```python
from build123d import *

# Parameters (mm, degrees)
SKETCH_1_R          = 2.75
EXTRUDE_1_DEPTH     = 3
FILLET_1_R          = 0.5
CUT_EXTRUDE_1_DEPTH = 2
SKETCH_3_R          = 1.5
EXTRUDE_2_DEPTH     = 8
CHAMFER_1_SIZE      = 0.2
FILLET_2_R          = 0.2


with BuildPart() as part:
    # 草图1 → 凸台-拉伸1 (new body)
    with BuildSketch(Plane.XY):
        Circle(SKETCH_1_R)
    extrude(amount=EXTRUDE_1_DEPTH)

    # 圆角1
    fillet_1_edges = [part.edges().sort_by_distance(p)[0] for p in [
        (-2.75, 0, 3),
    ]]
    fillet(fillet_1_edges, radius=FILLET_1_R)

    # 草图2 → 切除-拉伸1 (cut)
    with BuildSketch(Plane.XY.offset(3)):
        Polygon((1.558845727, 0), (0.779422863, 1.35), (-0.779422863, 1.35), (-1.558845727, 0), (-0.779422863, -1.35), (0.779422863, -1.35), align=None)
    extrude(amount=-CUT_EXTRUDE_1_DEPTH, mode=Mode.SUBTRACT)

    # 草图3 → 凸台-拉伸2 (add)
    with BuildSketch(Plane(origin=(0, 0, 0), x_dir=(-1, 0, 0), z_dir=(0, 0, -1))):
        Circle(SKETCH_3_R)
    extrude(amount=EXTRUDE_2_DEPTH)

    # 倒角1
    chamfer_1_edges = [part.edges().sort_by_distance(p)[0] for p in [
        (1.5, 0, -8),
    ]]
    chamfer(chamfer_1_edges, length=CHAMFER_1_SIZE)

    # 圆角2
    fillet_2_edges = [part.edges().sort_by_distance(p)[0] for p in [
        (-2.75, 0, 0),
    ]]
    fillet(fillet_2_edges, radius=FILLET_2_R)


solid = part.part
```
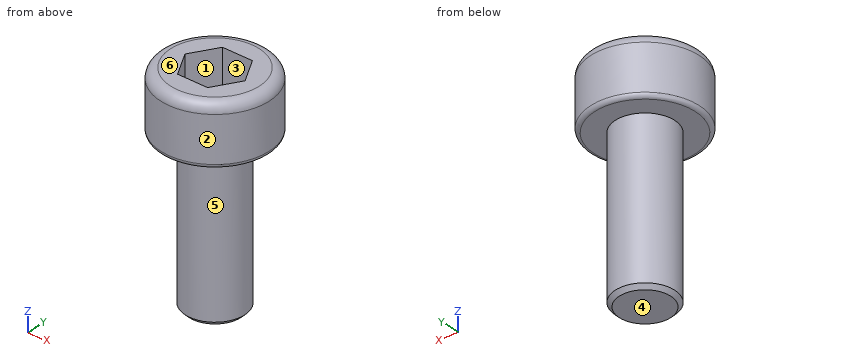
Input: part model. Units: mm. Frame: model coordinates. Face numbers are marked on the shaded views. A direction names the side the tool comes from. Coordinates: 2 decimals unless noted, no trailing zeros. Loops run counter-clockwise (first coordinate to the right, second up) from the corner with the lowest first, then second, coordinate; pieces in that order, holes last. Notation, with made-up numbers: M 3.25,20.25 L 34.25,20.25 A9 ccw 34.25,26.25 Z; hole C -19,24.25 d6. An arc over 180 degrees is marked long. Use a Markdown table: item, result. Add a question column.
1) Line query: L1, parallel to X at y = -0.75, z = -5.5; L2, parallel to Z at x = -0.9, y = -0.1. Output: solid intervals per line, ascending. Write a range as from..to.
2) Section A-A, the plane x = 0. Return the cut outline in (y, z), plus the area to 3 significant figures.
3) Section B-B, the plane z = -2. Return the cut outline in (x, y).
4) Draft query along X for the marked faces 1, 2, 3 and 4. Return one class per face: +X half, -X half, draft (parallel to the pull), parting line (faces both ways), or undercut.
5) Pin query (flat end, axial travel): P1, Ø1.7, axis at x = 0.5, z = 2, coming from the +Y side; P2, Ø0.5, axis at x = -0.5, z = 2, coming from the -Y side; P3, Ø2, axis at x = -1.5, z = -1.5, coming from the -Y side; P4, Ø1.5, axis at x = 0.5, z = -2.5, coming from the -Y side. Return the tip coordinate at first contact, or that it passes through.
6) Set-up query: the marked faces 5 and 6. Return all of +Z, -Z, +X, -X, +Y, -Y with unobstructed straight access to the full face (end or side cutting, diameter ignored); none if empty.
Answer below:
| question | item | result |
|---|---|---|
| 1 | L1 | -1.3..1.3 |
| 1 | L2 | -8..1 |
| 2 | outline | M -2.75,0.2 A0.2 ccw -2.55,0 L -1.5,0 L -1.5,-7.8 L -1.3,-8 L 1.3,-8 L 1.5,-7.8 L 1.5,0 L 2.55,0 A0.2 ccw 2.75,0.2 L 2.75,2.5 A0.5 ccw 2.25,3 L 1.35,3 L 1.35,1 L -1.35,1 L -1.35,3 L -2.25,3 A0.5 ccw -2.75,2.5 Z |
| 2 | area | 34.9 mm2 |
| 3 | outline | C 0,0 d3 |
| 4 | face 1 | undercut |
| 4 | face 2 | parting line |
| 4 | face 3 | undercut |
| 4 | face 4 | draft |
| 5 | P1 | y = 2.75 |
| 5 | P2 | y = -2.74 |
| 5 | P3 | y = -1.41 |
| 5 | P4 | y = -1.5 |
| 6 | face 5 | -Z |
| 6 | face 6 | +Z, +X, -X, +Y, -Y |
